The model under review builds one solid part; all positions refer to its coordinate system, in mm. Face numbers are marked on the shaded views. A direction names the side the tool comes from. Give positions to 0.01 mm unless a question says otherwise; leave off trailing zeros. Order: outer loops, then holes, each group sorted by start corner. A loop starts at its lowest first (then second) coordinate and runs counter-clockwise, first axis right, second up. Notation, with made-up numbers: (43.5, -9.75) - (87.5, -9.75) arc R22 ccw to (87.5, 13.25) - close; hole circle Ø2 at (15, 12.5). An arc over 180 degrees is marked (long way). Use CSV: the item, a comma, the result in double quotes.
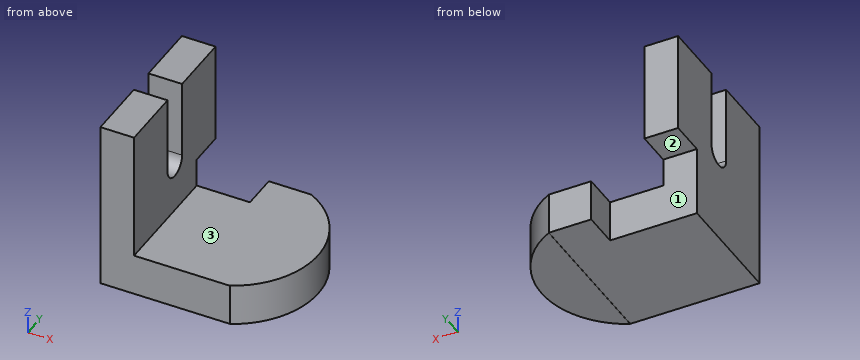
```python
from build123d import *

# Parameters (mm, degrees)
F1_DEPTH = 38.1
F3_DEPTH = 20.828
F4_W     = 13.647594
F4_H     = 2.408188
F5_DEPTH = 50.8
F6_W     = 26.398936
F6_H     = 17.6022
F7_DEPTH = 50.8
F9_DEPTH = 50.8


with BuildPart() as f1:
    # F0 (on Front) → F1 (new body, symmetric)
    with BuildSketch(Plane.XZ):
        Polygon((0, 38.717061), (-16.683353, 38.717061), (-16.683353, -46.183128), (47.443293, -46.183128), (47.443293, -25.435435), (0, -25.435435), align=None)
    extrude(amount=F1_DEPTH, both=True)

    # F2 (on face) → F3 (join)
    with BuildSketch(Plane.XY.offset(-25.435435)):
        with BuildLine():
            Line((47.443293, 38.1), (47.443293, -38.1))
            ThreePointArc((47.443293, -38.1), (71.140257, 0), (47.443293, 38.1))
        make_face()
    extrude(amount=-F3_DEPTH)

    # F4 (on face) → F5 (cut)
    with BuildSketch(Plane.YZ):
        with BuildLine():
            ThreePointArc((-6.823797, 0), (0, 6.823797), (6.823797, 0))
            Line((6.823797, 0), (6.823797, 38.717061))
            Line((6.823797, 38.717061), (-6.823797, 38.717061))
            Line((-6.823797, 38.717061), (-6.823797, 0))
        make_face()
        with Locations((0, 39.921155)):
            Rectangle(F4_W, F4_H)
        with BuildLine():
            Line((-6.823797, 0), (6.823797, 0))
            ThreePointArc((6.823797, 0), (0, 6.823797), (-6.823797, 0))
        make_face()
        with BuildLine():
            ThreePointArc((-6.823797, 0), (0, -6.823797), (6.823797, 0))
            Line((6.823797, 0), (-6.823797, 0))
        make_face()
    extrude(amount=-F5_DEPTH, mode=Mode.SUBTRACT)

    # F6 (on face) → F7 (cut)
    with BuildSketch(Plane.XY.offset(-25.435435)):
        with Locations((13.199468, 29.2989)):
            Rectangle(F6_W, F6_H)
    extrude(amount=-F7_DEPTH, mode=Mode.SUBTRACT)

    # F8 (on face) → F9 (cut)
    with BuildSketch(Plane.YZ):
        Polygon((20.4978, -11.306379), (20.4978, -25.435435), (20.4978, -46.183128), (38.1, -46.183128), (38.1, -11.306379), align=None)
    extrude(amount=-F9_DEPTH, mode=Mode.SUBTRACT)


solid = f1.part
```
Item 1: Take a section at A-A, the plane z = 2. Give the boundary of the cut face in (x, y), and give its area (3 significant figures).
Results list:
outline,"(-16.68, -38.1) - (0, -38.1) - (0, -6.82) - (-16.68, -6.82) - close; (-16.68, 6.82) - (0, 6.82) - (0, 38.1) - (-16.68, 38.1) - close"
area,"1,040 mm2"
Item 2: Take a section at D-D, the plane z = -40. Give the boundary of the cut face in (x, y), and give its area (3 significant figures).
Results list:
outline,"(-16.68, -38.1) - (47.44, -38.1) arc R42.48 ccw to (47.44, 38.1) - (26.4, 38.1) - (26.4, 20.5) - (-16.68, 20.5) - close"
area,"5,420 mm2"
Item 3: Take a section at B-B, the plane y = 0. Give the boundary of the cut face in (x, z).
Results list:
outline,"(-16.68, -46.18) - (47.44, -46.18) - (47.44, -46.26) - (71.14, -46.26) - (71.14, -25.44) - (0, -25.44) - (0, -6.82) - (-16.68, -6.82) - close"
Item 4: Wall thickness on L1, parallel to Y at x = -12, z = 16; L2, parallel to Z at x = 61, y = 17.5; L3, parallel to X at y = -16, z = -13: over which ranges is each line inside the solid? List them lowest first.
Results list:
L1,"y = -38.1 to -6.82, 6.82 to 38.1"
L2,"z = -46.26 to -25.44"
L3,"x = -16.68 to 0"
Item 5: Tool access review of the marked faces 1, 2 and 3: name each direction out of +Z, -Z, +X, -X, +Y, -Y from which nothing blocks a thin tool from reaching the whole face with its end or side.
Results list:
face 1,"-Z, -X, +Y"
face 2,"-Z, +X, -X, +Y"
face 3,"+Z, +X, +Y, -Y"
Item 6: Take a section at C-C, the plane y = 32.5. Give the boundary of the cut face in (x, z).
Results list:
outline,"(-16.68, -11.31) - (0, -11.31) - (0, 38.72) - (-16.68, 38.72) - close; (26.4, -46.18) - (47.44, -46.18) - (47.44, -46.26) - (56.01, -46.26) - (56.01, -25.44) - (26.4, -25.44) - close"
Item 7: Clearance check with flat-ended pins moving along their axes: pin 1 (6 mm diameter, centred on x = 42, y = -2.5, fed in from +Z); pin 2 (8.5 mm diameter, centred on x = -8, y = 26.5, fed in from -Z); pin 3 (9 mm diameter, centred on y = 33, z = -34, fed in from -X). State where each tip first meets the part, or that it passes through.
Results list:
pin 1,"stops at z = -25.44"
pin 2,"stops at z = -11.31"
pin 3,"stops at x = 26.4"
